The listing builds one solid part. Answer for the finished solid, in the listing's coordinates (mm). Face numbers are marked on the shaded views. A direction names the side the tool comes from. Round coordinates to 2 decimals unless told otherwise and drop trailing zeros. Loops run counter-clockwise (first coordinate to the right, second up) from the corner with the lowest first, then second, coordinate; pieces in that order, holes last. Notation, with made-up numbers: M 47,27.25 L 60,27.25 A29 cw 60,50.25 Z; hole C -4.75,43 d8. An arc over 180 degrees is marked long. Put each result on its own line as item: value. Start each with the question number.
(1) Section C-C, the plane z = 0 is taken. Determine the outline of the cut face in (x, y).
(2) Determine the mould class of the marked faces 1, 2 and 3 for opening direction X: released by +X, released by -X, zero draft, split by the parting line, or undercut.
(3) Flat-ended cylindrical pins translate along their axes: P1, Ø3, axis at x = -27, y = 10.5, coming from the +Z side; P2, Ø4, axis at y = 7.5, z = -27, coming from the -X side; P3, Ø3, axis at x = 59, z = -30, coming from the +Y side. Find the tip coordinate at first contact, or state that the pin passes through.
(4) Section B-B, the plane x = 0 is taken. Determine the outline of the cut face in (y, z), then the cut area to 3 significant figures.
(5) Section A-A, the plane y = 10.25 is taken. Determine the outline of the cut face in (x, z).
(6) Straight lines are drawn through the part: line 1 (Y direction, x = 43, z = 22.5); line 2 (X direction, y = 10.2, z = 48); line 3 (Z direction, x = -35.5, y = 8.5). For each, find the intervals that lie inside material, in ascending order.
(7) Which of the six approach directions +Z, -Z, +X, -X, +Y, -Y give full straight-line access (tool end or side, diameter ignored) to the marked faces 4 and 5?
```python
from build123d import *

# Parameters (mm, degrees)
ESQUISSE1_R             = 76.3
BOSS_EXTRU_1_DEPTH      = 12
CONG_1_R                = 12.7
ESQUISSE2_R             = 10
ESQUISSE2_R_2           = 10.5
ENL_V_MAT_EXTRU_1_DEPTH = 5


with BuildPart() as part:
    # Esquisse1 → Boss.-Extru.1 (new body)
    with BuildSketch(Plane(origin=(0, 0, 0), x_dir=(1, 0, 0), z_dir=(0, 1, 0))):
        with Locations(Location((0, 0, 0), (0, 0, 270))):
            Circle(ESQUISSE1_R)
    extrude(amount=BOSS_EXTRU_1_DEPTH)

    # Congé1
    # the kernel refuses this fillet: 12.7 mm, written as the material it takes off along each edge
    with BuildSketch(Plane(origin=(0, 12, 0), x_dir=(0, 0, 1), z_dir=(-1, 0, 0))) as cong_1_piece_1:
        with BuildLine():
            CenterArc((63.619306013, -12.7), CONG_1_R, 3.159636303, 86.840363697)
            Line((63.619306013, 0), (63.619306013, 0.254))
            Line((63.619306013, 0.254), (76.3, 0.254))
            Line((76.3, 0.254), (76.554, 0))
            ThreePointArc((76.554, 0), (76.554, -6), (76.55361388, -11.986))
            Line((76.55361388, -11.986), (76.3, -12))
        make_face()
    revolve(axis=Axis((0, 12, 0), (0, 1, 0)), mode=Mode.SUBTRACT)

    # Esquisse2 → Enlèv. mat.-Extru.1 (cut)
    with BuildSketch(Plane(origin=(0, 12, 0), x_dir=(1, 0, 0), z_dir=(0, 1, 0))):
        with Locations(Location((0, 0, 0), (0, 0, 270))):
            Circle(ESQUISSE2_R)
        with Locations(Location((0, 48, 0), (0, 0, 270))):
            Circle(ESQUISSE2_R_2)
        with Locations(Location((41.569219382, 24, 0), (0, 0, 270))):
            Circle(ESQUISSE2_R_2)
        with Locations(Location((41.569219382, -24, 0), (0, 0, 270))):
            Circle(ESQUISSE2_R_2)
        with Locations(Location((0, -48, 0), (0, 0, 270))):
            Circle(ESQUISSE2_R_2)
        with Locations(Location((-41.569219382, -24, 0), (0, 0, 270))):
            Circle(ESQUISSE2_R_2)
        with Locations(Location((-41.569219382, 24, 0), (0, 0, 270))):
            Circle(ESQUISSE2_R_2)
    extrude(amount=-ENL_V_MAT_EXTRU_1_DEPTH, mode=Mode.SUBTRACT)


solid = part.part
```
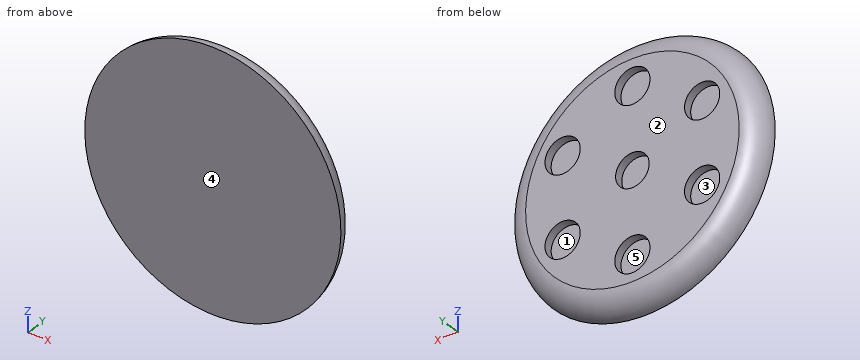
Recorded:
1. outline: M -76.3,0 L 76.3,0 A12.7 ccw 63.62,12 L 10,12 L 10,7 L -10,7 L -10,12 L -63.62,12 A12.7 ccw Z
2. face 1: undercut
2. face 2: zero draft
2. face 3: undercut
3. P1: stops at z = 66.64
3. P2: stops at x = -69.87
3. P3: stops at y = 11.95
4. outline: M 0,-76.3 A12.7 ccw 12,-63.62 L 12,-58.5 L 7,-58.5 L 7,-37.5 L 12,-37.5 L 12,-10 L 7,-10 L 7,10 L 12,10 L 12,37.5 L 7,37.5 L 7,58.5 L 12,58.5 L 12,63.62 A12.7 ccw 0,76.3 Z
4. area: 1,450 mm²
5. outline: C 0,0 d140.11; hole C -41.57,-24 d21; hole C -41.57,24 d21; hole C 0,-48 d21; hole C 0,48 d21; hole C 0,0 d20; hole C 41.57,-24 d21; hole C 41.57,24 d21
6. line 1: y = 0 to 7
6. line 2: x = -51.14 to -10.5, 10.5 to 51.14
6. line 3: z = -63.07 to -32.57, -15.43 to 15.43, 32.57 to 63.07
7. face 4: +Z, -Z, +X, -X, -Y
7. face 5: +Y
